```python
from build123d import *

# Parameters (mm, degrees)
F1_DEPTH = 1.5875


# Not quite as in the source:
# - a length typed as a fraction of an inch, garbled in the dataset ("3 / 203.2 mm" for 3/8 in), is restored


with BuildPart() as f1:
    # F0 (on Top) → F1 (new body)
    with BuildSketch(Plane.XY):
        with BuildLine():
            Line((22.098, 26.5938), (22.098, 31.115))
            Line((22.098, 31.115), (0, 31.115))
            Line((0, 31.115), (-22.098, 31.115))
            Line((-22.098, 31.115), (-22.098, 26.5938))
            ThreePointArc((-22.098, 26.5938), (-20.6252379961, 25.9837620039), (-20.0152, 24.511))
            ThreePointArc((-20.0152, 24.511), (-20.6252379961, 23.0382379961), (-22.098, 22.4282))
            Line((-22.098, 22.4282), (-22.098, 0.127))
            ThreePointArc((-22.098, 0.127), (-20.8407641431, -0.3937641431), (-20.32, -1.651))
            ThreePointArc((-20.32, -1.651), (-20.8407641431, -2.9082358569), (-22.098, -3.429))
            Line((-22.098, -3.429), (-22.098, -9.779))
            Line((-22.098, -9.779), (22.098, -9.779))
            Line((22.098, -9.779), (22.098, -3.7338))
            ThreePointArc((22.098, -3.7338), (20.0152, -1.651), (22.098, 0.4318))
            Line((22.098, 0.4318), (22.098, 22.4282))
            ThreePointArc((22.098, 22.4282), (20.0152, 24.511), (22.098, 26.5938))
        make_face()
        with BuildLine():
            Line((-22.098, 26.5938), (-22.098, 31.115))
            Line((-22.098, 31.115), (-33.02, 31.115))
            Line((-33.02, 31.115), (-33.02, -31.115))
            Line((-33.02, -31.115), (-22.098, -31.115))
            Line((-22.098, -31.115), (-22.098, -27.559))
            Line((-22.098, -27.559), (-22.098, -19.939))
            Line((-22.098, -19.939), (-22.098, -9.779))
            Line((-22.098, -9.779), (-22.098, -3.429))
            ThreePointArc((-22.098, -3.429), (-23.876, -1.651), (-22.098, 0.127))
            Line((-22.098, 0.127), (-22.098, 22.4282))
            ThreePointArc((-22.098, 22.4282), (-24.1808, 24.511), (-22.098, 26.5938))
        make_face()
        with BuildLine():
            Line((33.02, -27.559), (33.02, 31.115))
            Line((33.02, 31.115), (22.098, 31.115))
            Line((22.098, 31.115), (22.098, 26.5938))
            ThreePointArc((22.098, 26.5938), (23.5707620039, 25.9837620039), (24.1808, 24.511))
            ThreePointArc((24.1808, 24.511), (23.5707620039, 23.0382379961), (22.098, 22.4282))
            Line((22.098, 22.4282), (22.098, 0.4318))
            ThreePointArc((22.098, 0.4318), (23.5707620039, -0.1782379961), (24.1808, -1.651))
            ThreePointArc((24.1808, -1.651), (23.5707620039, -3.1237620039), (22.098, -3.7338))
            Line((22.098, -3.7338), (22.098, -9.779))
            Line((22.098, -9.779), (22.098, -19.939))
            Line((22.098, -19.939), (22.098, -27.559))
            Line((22.098, -27.559), (23.9649, -27.559))
            ThreePointArc((23.9649, -27.559), (26.0477, -25.4762), (28.1305, -27.559))
            Line((28.1305, -27.559), (33.02, -27.559))
        make_face()
        with BuildLine():
            Line((33.02, -31.115), (33.02, -27.559))
            Line((33.02, -27.559), (28.1305, -27.559))
            ThreePointArc((28.1305, -27.559), (26.0477, -29.6418), (23.9649, -27.559))
            Line((23.9649, -27.559), (22.098, -27.559))
            Line((22.098, -27.559), (22.098, -31.115))
            Line((22.098, -31.115), (33.02, -31.115))
        make_face()
        with BuildLine():
            Line((-14.4272, -27.559), (22.098, -27.559))
            Line((22.098, -27.559), (22.098, -19.939))
            Line((22.098, -19.939), (-22.098, -19.939))
            Line((-22.098, -19.939), (-22.098, -27.559))
            Line((-22.098, -27.559), (-18.5928, -27.559))
            ThreePointArc((-18.5928, -27.559), (-16.51, -25.4762), (-14.4272, -27.559))
        make_face()
        with BuildLine():
            Line((-22.098, -31.115), (22.098, -31.115))
            Line((22.098, -31.115), (22.098, -27.559))
            Line((22.098, -27.559), (-14.4272, -27.559))
            ThreePointArc((-14.4272, -27.559), (-16.51, -29.6418), (-18.5928, -27.559))
            Line((-18.5928, -27.559), (-22.098, -27.559))
            Line((-22.098, -27.559), (-22.098, -31.115))
        make_face()
    extrude(amount=F1_DEPTH)


solid = f1.part
```
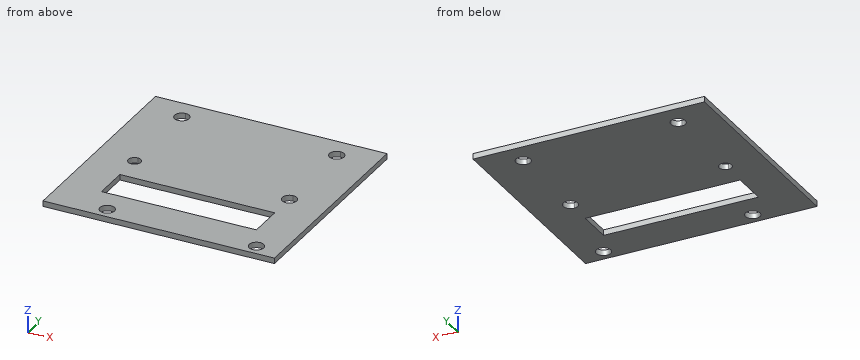
Check sheet for the modelled part. Datum: model origin and axes. Units: mm. Coordinates: 2 decimals unless noted, no trailing zeros. Write each loop counter-clockwise with the first axis right and the second up, starting at its lowest first coordinate (ties: lowest second). Pieces come first, ordered by that corner, then holes. Notation, with made-up numbers: (-0.5, -19.75) -> (37.5, -19.75) arc R27 cw to (37.5, 14.25) -> close; hole circle Ø7 at (-14.75, 41). An arc over 180 degrees is marked (long way). Use a Markdown table: item, result.
1. Sectioned sample at C-C (x = -16.51). Enter the section's corners in (y, z) (1 decimal).
Reported:
| item | result |
|---|---|
| outline | (-31.1, 0) -> (-29.6, 0) -> (-29.6, 1.6) -> (-31.1, 1.6) -> close; (-25.5, 0) -> (-19.9, 0) -> (-19.9, 1.6) -> (-25.5, 1.6) -> close; (-9.8, 0) -> (31.1, 0) -> (31.1, 1.6) -> (-9.8, 1.6) -> close |
2. Sectioned sample at B-B (y = -11.5). Enter the section's corners in (x, z).
Reported:
| item | result |
|---|---|
| outline | (-33.02, 0) -> (-22.1, 0) -> (-22.1, 1.59) -> (-33.02, 1.59) -> close; (22.1, 0) -> (33.02, 0) -> (33.02, 1.59) -> (22.1, 1.59) -> close |
3. Sectioned sample at D-D (z = 1.1). Enter the section's corners in (x, y) (3 decimals).
Reported:
| item | result |
|---|---|
| outline | (-33.02, -31.115) -> (33.02, -31.115) -> (33.02, 31.115) -> (-33.02, 31.115) -> close; hole circle Ø4.166 at (-22.098, 24.511); hole circle Ø3.556 at (-22.098, -1.651); hole (-22.098, -19.939) -> (22.098, -19.939) -> (22.098, -9.779) -> (-22.098, -9.779) -> close; hole circle Ø4.166 at (-16.51, -27.559); hole circle Ø4.166 at (22.098, -1.651); hole circle Ø4.166 at (22.098, 24.511); hole circle Ø4.166 at (26.048, -27.559) |
4. Scan lines: line 1 along Y through (x, z) = (-16.51, 0.9) (3 decimals); line 2 along X through (y, z) = (-10.5, 0.85); line 3 along Y through (x, z) = (-22, 0.9) (1 decimal). Record each from-to range of solid material in increasing order.
Reported:
| item | result |
|---|---|
| line 1 | y = -31.115 to -29.642, -25.476 to -19.939, -9.779 to 31.115 |
| line 2 | x = -33.02 to -22.1, 22.1 to 33.02 |
| line 3 | y = -31.1 to -19.9, -9.8 to -3.4, 0.1 to 22.4, 26.6 to 31.1 |
5. Sectioned sample at A-A (x = 14). Enter the section's corners in (y, z) (1 decimal), plus the area to 3 significant figures.
Reported:
| item | result |
|---|---|
| outline | (-31.1, 0) -> (-19.9, 0) -> (-19.9, 1.6) -> (-31.1, 1.6) -> close; (-9.8, 0) -> (31.1, 0) -> (31.1, 1.6) -> (-9.8, 1.6) -> close |
| area | 82.7 mm2 |
6. Go/stop test with a flat-tipped pin: pin 1 Ø10 at (x, y) = (3.5, -15.5) entering from -Z. Record where the tip stops, or that it passes through.
Reported:
| item | result |
|---|---|
| pin 1 | stops at z = 0 |
